Build history of the part. All positions in model axes, mm. Face numbers are marked on the shaded views. A direction names the side the tool comes from. Round coordinates to 2 decimals unless told otherwise and drop trailing zeros. Loops run counter-clockwise (first coordinate to the right, second up) from the corner with the lowest first, then second, coordinate; pieces in that order, holes last. Notation, with made-up numbers: M 48,13.5 L 66,13.5 A11 ccw 66,27.5 Z; hole C 56.5,65 d11. An arc over 180 degrees is marked long. Write each question's results on one line, items separated by ' | '. Start each with the question number.
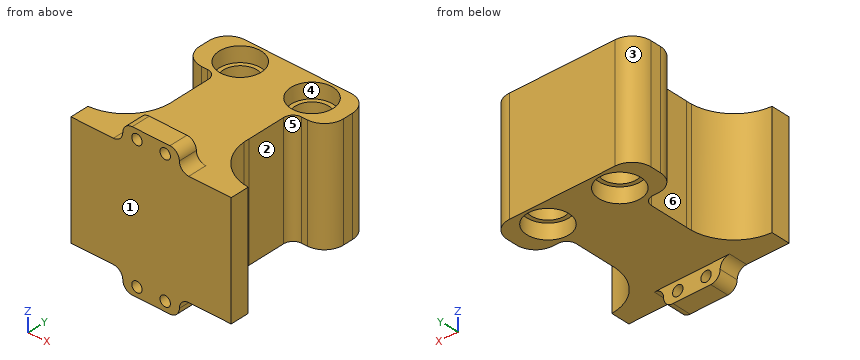
```python
from build123d import *

# Parameters (mm, degrees)
SKETCH1_W           = 15
SKETCH1_H           = 10
SKETCH1_R           = 2.75
SKETCH1_W_2         = 85
SKETCH1_H_2         = 60
BOSS_EXTRUDE1_DEPTH = 10
BOSS_EXTRUDE2_DEPTH = 70
CUT_EXTRUDE1_DEPTH  = 10
FILLET1_START       = -1
FILLET1_DEPTH       = 11
FILLET1_2_DEPTH     = 10
SKETCH5_R           = 9
BOSS_EXTRUDE3_DEPTH = 60
SKETCH6_R           = 11.15
CUT_EXTRUDE2_DEPTH  = 8
CUT_EXTRUDE3_START  = -8
SKETCH7_R           = 11.15
CUT_EXTRUDE3_DEPTH  = 8
FILLET2_R           = 10
FILLET3_R           = 5


with BuildPart() as part:
    # Sketch1 → Boss-Extrude1 (new body)
    # profile 1 of 5: a face of its own
    with BuildSketch(Plane(origin=(0, 0, 0), x_dir=(1, 0, 0), z_dir=(0, 1, 0))):
        with Locations((35, 65)):
            Rectangle(SKETCH1_W, SKETCH1_H)
        with Locations(Location((35, 65, 0), (0, 0, 270))):
            Circle(SKETCH1_R, mode=Mode.SUBTRACT)
    # profile 2 of 5: a face of its own
    with BuildSketch(Plane(origin=(0, 0, 0), x_dir=(1, 0, 0), z_dir=(0, 1, 0))):
        with Locations((50, 65)):
            Rectangle(SKETCH1_W, SKETCH1_H)
        with Locations(Location((50, 65, 0), (0, 0, 270))):
            Circle(SKETCH1_R, mode=Mode.SUBTRACT)
    # profile 3 of 5: a face of its own
    with BuildSketch(Plane(origin=(0, 0, 0), x_dir=(1, 0, 0), z_dir=(0, 1, 0))):
        with Locations((50, -5)):
            Rectangle(SKETCH1_W, SKETCH1_H)
        with Locations(Location((50, -5, 0), (0, 0, 270))):
            Circle(SKETCH1_R, mode=Mode.SUBTRACT)
    # profile 4 of 5: a face of its own
    with BuildSketch(Plane(origin=(0, 0, 0), x_dir=(1, 0, 0), z_dir=(0, 1, 0))):
        with Locations((35, -5)):
            Rectangle(SKETCH1_W, SKETCH1_H)
        with Locations(Location((35, -5, 0), (0, 0, 270))):
            Circle(SKETCH1_R, mode=Mode.SUBTRACT)
    # profile 5 of 5: a face of its own
    with BuildSketch(Plane(origin=(0, 0, 0), x_dir=(1, 0, 0), z_dir=(0, 1, 0))):
        with Locations((42.5, 30)):
            Rectangle(SKETCH1_W_2, SKETCH1_H_2)
    extrude(amount=BOSS_EXTRUDE1_DEPTH)

    # Sketch4 → Boss-Extrude2 (add)
    with BuildSketch(Plane(origin=(0, 0, -70), x_dir=(-1, 0, 0), z_dir=(0, 0, -1))):
        with BuildLine():
            Line((-85, 10), (-62.5, 10))
            Line((-62.5, 10), (-62.5, 32.5))
            ThreePointArc((-62.5, 32.5), (-69.483783569, 16.983783569), (-85, 10))
        make_face()
        with BuildLine():
            Line((-57.5, 10), (-42.5, 10))
            Line((-42.5, 10), (-42.5, 60.8))
            Line((-42.5, 60.8), (-62.5, 60.8))
            Line((-62.5, 60.8), (-62.5, 35.4))
            ThreePointArc((-62.5, 35.4), (-62.45614662, 33.95), (-62.5, 32.5))
            Line((-62.5, 32.5), (-62.5, 10))
            Line((-62.5, 10), (-57.5, 10))
        make_face()
        with BuildLine():
            Line((-42.5, 60.8), (-42.5, 10))
            Line((-42.5, 10), (-27.5, 10))
            Line((-27.5, 10), (-22.5, 10))
            Line((-22.5, 10), (-22.5, 32.5))
            ThreePointArc((-22.5, 32.5), (-22.54385338, 33.95), (-22.5, 35.4))
            Line((-22.5, 35.4), (-22.5, 60.8))
            Line((-22.5, 60.8), (-42.5, 60.8))
        make_face()
        with BuildLine():
            Line((-22.5, 32.5), (-22.5, 10))
            Line((-22.5, 10), (0, 10))
            ThreePointArc((0, 10), (-15.516216431, 16.983783569), (-22.5, 32.5))
        make_face()
    extrude(amount=-BOSS_EXTRUDE2_DEPTH)

    # Sketch4<4> → Cut-Extrude1 (cut)
    with BuildSketch(Plane(origin=(0, 0, -70), x_dir=(-1, 0, 0), z_dir=(0, 0, -1))):
        with BuildLine():
            Line((-57.5, 10), (-42.5, 10))
            Line((-42.5, 10), (-42.5, 60.8))
            Line((-42.5, 60.8), (-62.5, 60.8))
            Line((-62.5, 60.8), (-62.5, 35.4))
            ThreePointArc((-62.5, 35.4), (-62.45614662, 33.95), (-62.5, 32.5))
            Line((-62.5, 32.5), (-62.5, 10))
            Line((-62.5, 10), (-57.5, 10))
        make_face()
        with BuildLine():
            Line((-42.5, 60.8), (-42.5, 10))
            Line((-42.5, 10), (-27.5, 10))
            Line((-27.5, 10), (-22.5, 10))
            Line((-22.5, 10), (-22.5, 32.5))
            ThreePointArc((-22.5, 32.5), (-22.54385338, 33.95), (-22.5, 35.4))
            Line((-22.5, 35.4), (-22.5, 60.8))
            Line((-22.5, 60.8), (-42.5, 60.8))
        make_face()
        with BuildLine():
            Line((-85, 10), (-62.5, 10))
            Line((-62.5, 10), (-62.5, 32.5))
            ThreePointArc((-62.5, 32.5), (-69.483783569, 16.983783569), (-85, 10))
        make_face()
        with BuildLine():
            Line((-22.5, 32.5), (-22.5, 10))
            Line((-22.5, 10), (0, 10))
            ThreePointArc((0, 10), (-15.516216431, 16.983783569), (-22.5, 32.5))
        make_face()
    extrude(amount=-CUT_EXTRUDE1_DEPTH, mode=Mode.SUBTRACT)

    # Fillet1: read off the stored shape, not the designer's step
    # Fillet1 outline → Fillet1 (cut)
    with BuildSketch(Plane(origin=(0, 0, 0), x_dir=(1, 0, 0), z_dir=(0, 1, 0)).offset(FILLET1_START)):
        with BuildLine():
            Line((27.5, 70), (27.5, 65))
            ThreePointArc((27.5, 65), (28.964466094, 68.535533906), (32.5, 70))
            Line((32.5, 70), (27.5, 70))
        make_face()
        with BuildLine():
            Line((57.5, 70), (52.5, 70))
            ThreePointArc((52.5, 70), (56.035533906, 68.535533906), (57.5, 65))
            Line((57.5, 65), (57.5, 70))
        make_face()
        with BuildLine():
            Line((57.5, -10), (57.5, -5))
            ThreePointArc((57.5, -5), (56.035533906, -8.535533906), (52.5, -10))
            Line((52.5, -10), (57.5, -10))
        make_face()
        with BuildLine():
            Line((27.5, -10), (32.5, -10))
            ThreePointArc((32.5, -10), (28.964466094, -8.535533906), (27.5, -5))
            Line((27.5, -5), (27.5, -10))
        make_face()
    extrude(amount=FILLET1_DEPTH, mode=Mode.SUBTRACT)

    # Fillet1 2 outline → Fillet1 2 (add)
    with BuildSketch(Plane(origin=(0, 0, 0), x_dir=(1, 0, 0), z_dir=(0, 1, 0))):
        with BuildLine():
            ThreePointArc((27.5, 65), (26.035533906, 61.464466094), (22.5, 60))
            Line((22.5, 60), (27.5, 60))
            Line((27.5, 60), (27.5, 65))
        make_face()
        with BuildLine():
            Line((57.5, 65), (57.5, 60))
            Line((57.5, 60), (62.5, 60))
            ThreePointArc((62.5, 60), (58.964466094, 61.464466094), (57.5, 65))
        make_face()
        with BuildLine():
            Line((57.5, 0), (57.5, -5))
            ThreePointArc((57.5, -5), (58.964466094, -1.464466094), (62.5, 0))
            Line((62.5, 0), (57.5, 0))
        make_face()
        with BuildLine():
            Line((27.5, -5), (27.5, 0))
            Line((27.5, 0), (22.5, 0))
            ThreePointArc((22.5, 0), (26.035533906, -1.464466094), (27.5, -5))
        make_face()
    extrude(amount=FILLET1_2_DEPTH)

    # Sketch5 → Boss-Extrude3 (add)
    # profile 1 of 2: a face of its own
    with BuildSketch(Plane.XY):
        Polygon((22.5, 60.8), (42.5, 60.8), (42.5, 86.2), (4.4, 86.2), (4.4, 60.8), align=None)
        with Locations((23.45, 73.5)):
            Circle(SKETCH5_R, mode=Mode.SUBTRACT)
    # profile 2 of 2: a face of its own
    with BuildSketch(Plane.XY):
        Polygon((42.5, 86.2), (42.5, 60.8), (62.5, 60.8), (80.6, 60.8), (80.6, 86.2), align=None)
        with Locations((61.55, 73.5)):
            Circle(SKETCH5_R, mode=Mode.SUBTRACT)
    extrude(amount=-BOSS_EXTRUDE3_DEPTH)

    # Sketch6 → Cut-Extrude2 (cut)
    with BuildSketch(Plane.XY):
        with Locations((23.45, 73.5)):
            Circle(SKETCH6_R)
        with Locations((61.55, 73.5)):
            Circle(SKETCH6_R)
    extrude(amount=-CUT_EXTRUDE2_DEPTH, mode=Mode.SUBTRACT)

    # Sketch7 → Cut-Extrude3 (cut)
    with BuildSketch(Plane(origin=(0, 0, -60), x_dir=(-1, 0, 0), z_dir=(0, 0, -1)).offset(CUT_EXTRUDE3_START)):
        with Locations(Location((-61.55, 73.5, 0), (0, 0, 180))):
            Circle(SKETCH7_R)
        with Locations(Location((-23.45, 73.5, 0), (0, 0, 180))):
            Circle(SKETCH7_R)
    extrude(amount=CUT_EXTRUDE3_DEPTH, mode=Mode.SUBTRACT)

    # Fillet2
    fillet2_edges = [part.edges().sort_by_distance(p)[0] for p in [
        (80.6, 60.8, -30),
        (4.4, 60.8, -30),
        (4.4, 86.2, -30),
        (80.6, 86.2, -30),
    ]]
    fillet(fillet2_edges, radius=FILLET2_R)

    # Fillet3
    fillet3_edges = [part.edges().sort_by_distance(p)[0] for p in [
        (62.5, 60.8, -30),
        (22.5, 60.8, -30),
    ]]
    fillet(fillet3_edges, radius=FILLET3_R)


solid = part.part
```
Item 1: Mould opens along Y. For the marked faces 1, 2 and 3 say: released by +Y, released by -Y, zero draft, split by the parting line, or undercut.
Item 2: Saw through at B-B, the plane x = 74. Give the cut face in (y, z), then the cut area to 3 significant figures.
Item 3: Drop flat-ended pins along their axis: pin 1 (8 mm diameter, centred on x = 48, z = 5, fed in from +Y); pin 2 (10 mm diameter, centred on x = 26.5, y = 19, fed in from +Z); pin 3 (4.5 mm diameter, centred on x = 35, z = -65, fed in from +Y); pin 4 (3.5 mm diameter, centred on x = 69.5, z = -33.5, fed in from -Y). Give the stop position or say it passes through.
Item 4: Tool access for the marked faces 4, 5 and 6: list every direction of +Z, -Z, +X, -X, +Y, -Y with a clear straight run to the whole face (end or side of a thin tool).
Item 5: Drill centre lines: line 1 along X through (y, z) = (73, -2); line 2 along Y through (x, z) = (61.55, -5.75); line 3 along Y through (x, z) = (61, -39). Where is each one in solid material? Low to high. Write a range as [from, to].
Item 6: Saw through at A-A, the plane y = 73.5. Give the cut face in (x, z).
Item 7: Saw through at D-D, the plane x = 45.5. Give the cut face in (y, z).
Item 8: Saw through at C-C, the plane z = -47.5. Give the cut face in (x, y).
Working result:
1) face 1: released by -Y | face 2: undercut | face 3: released by +Y
2) outline: M 0,-60 L 13.44,-60 L 13.44,0 L 0,0 Z; M 61.4,-60 L 85.6,-60 L 85.6,0 L 61.4,0 Z | area: 2,260 mm²
3) pin 1: stops at y = 10 | pin 2: stops at z = 0 | pin 3: passes through | pin 4: stops at y = 0
4) face 4: +Z | face 5: +Z, -Z, +X | face 6: +Z, -Z, -X
5) line 1: x = [4.4, 12.31], [34.59, 50.41], [72.69, 80.6] | line 2: y = [0, 62.35], [84.65, 86.2] | line 3: y = [0, 64.52], [82.48, 86.2]
6) outline: M 4.4,-60 L 12.3,-60 L 12.3,-52 L 14.45,-52 L 14.45,-8 L 12.3,-8 L 12.3,0 L 4.4,0 Z; M 32.45,-52 L 34.6,-52 L 34.6,-60 L 50.4,-60 L 50.4,-52 L 52.55,-52 L 52.55,-8 L 50.4,-8 L 50.4,0 L 34.6,0 L 34.6,-8 L 32.45,-8 Z; M 70.55,-52 L 72.7,-52 L 72.7,-60 L 80.6,-60 L 80.6,0 L 72.7,0 L 72.7,-8 L 70.55,-8 Z
7) outline: M 0,-70 L 10,-70 L 10,-60 L 86.2,-60 L 86.2,0 L 10,0 L 10,10 L 0,10 Z
8) outline: M 0,0 L 85,0 L 85,10 A23.99 cw 62.5,35.4 L 62.5,55.8 A5 cw 67.5,60.8 L 70.6,60.8 A10 ccw 80.6,70.8 L 80.6,76.2 A10 ccw 70.6,86.2 L 14.4,86.2 A10 ccw 4.4,76.2 L 4.4,70.8 A10 ccw 14.4,60.8 L 17.5,60.8 A5 cw 22.5,55.8 L 22.5,35.4 A23.99 cw 0,10 Z; hole C 23.45,73.5 d18; hole C 61.55,73.5 d18
